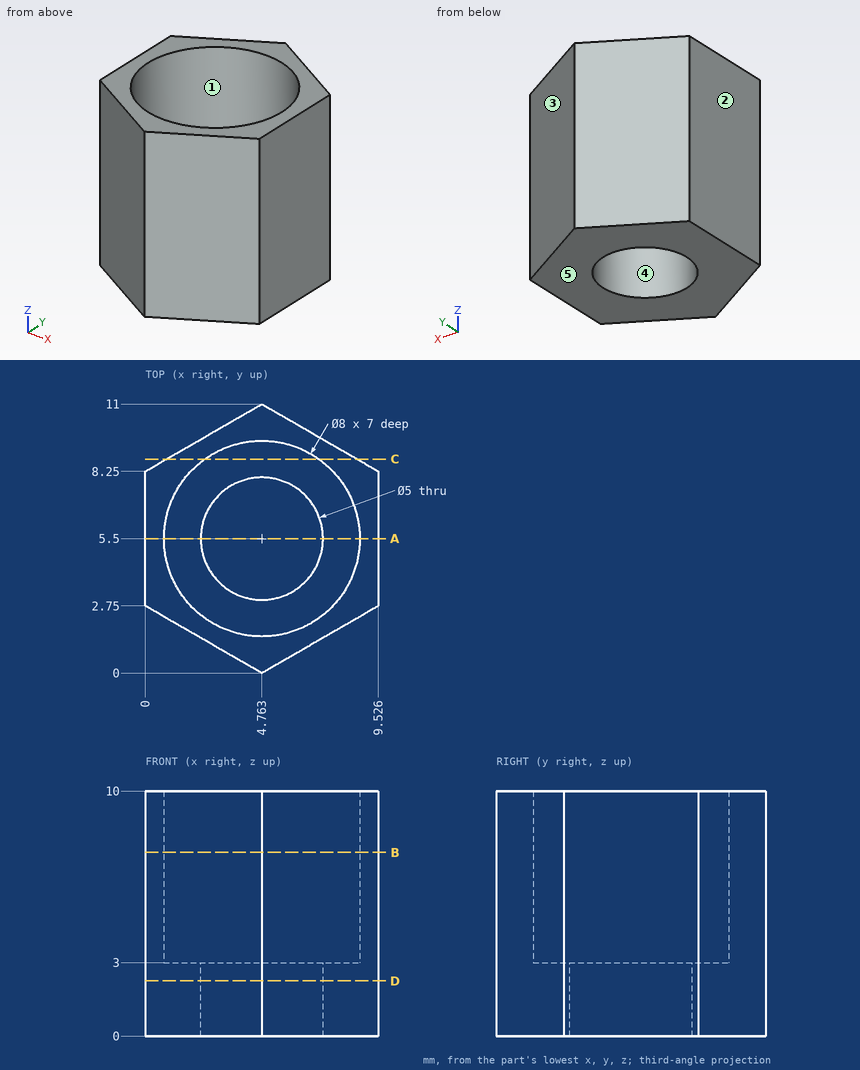
Design review of the part shown in the three views and the two pictorial views. Dimensions are in mm from the part's minimum x, y and z. A direction names the side the tool comes from. Give positions to 0.01 mm unless a question says otherwise; leave off trailing zeros. Write each loop counter-clockwise with the first axis right and the second up, starting at its lowest first coordinate (ties: lowest second). Pieces come first, ordered by that corner, then holes. Notation, with made-up numbers: (-33.5, 11.25) - (18.5, 11.25) arc R13 cw to (18.5, 31.25) - close; hole circle Ø9 at (8, 87.5). An arc over 180 degrees is marked (long way). Return JSON: item names as keys, results as strings. Group by question number.
(1) We need section B-B, the plane z = 7.5. Give the boundary of the cut face in (x, y).
(2) Machinability: for the marked faces 1 and 2, which of the approach directions +Z, -Z, +X, -X, +Y, -Y give a long, thin tool a straight path to every point of the face, cutting with its end or side? Answer none if there is none.
(3) We need section A-A, the plane y = 5.5. Give the boundary of the cut face in (x, z).
(4) Mouldability with a two-part tool opening along Y and no side actions: class the marked faces 3, 4 and 5 as +Y half, -Y half, draft (parallel to the pull), parting line (faces both ways), or undercut.
(5) We need section C-C, the plane y = 8.75. Give the boundary of the cut face in (x, z) (1 decimal).
(6) Insertion check: pin 1 (1 mm diameter, centred on y = 1, z = 4.5, fed in from -X) (1 decimal); pin 2 (1 mm diameter, centred on x = 7.5, y = 5, fed in from +Z); pin 3 (4 mm diameter, centred on x = 4.5, z = 6, fed in from +Y). Each pin has a flat end and moves straight along its axis. Give the tip position at first contact, or say it passes through.
(7) We need section D-D, the plane z = 2.25. Give the boundary of the cut face in (x, y).
(8) To check wall thickness, follow probe 1 along X at (y, z) = (5.5, 0.8); probe 2 along X at (y, z) = (5.5, 6.5); probe 3 along Z at (x, y) = (2.25, 4.25). State the ranges of each line that lie inside material, in increasing order.
Reported:
{
 "1": {"outline": "(0, 2.75) - (4.76, 0) - (9.53, 2.75) - (9.53, 8.25) - (4.76, 11) - (0, 8.25) - close; hole circle Ø8 at (4.76, 5.5)"},
 "2": {"face 1": "+Z", "face 2": "+Z, -Z, -X, +Y, -Y"},
 "3": {"outline": "(0, 0) - (2.26, 0) - (2.26, 3) - (0.76, 3) - (0.76, 10) - (0, 10) - close; (7.26, 0) - (9.53, 0) - (9.53, 10) - (8.76, 10) - (8.76, 3) - (7.26, 3) - close"},
 "4": {"face 3": "+Y half", "face 4": "undercut", "face 5": "draft"},
 "5": {"outline": "(0.9, 0) - (8.7, 0) - (8.7, 10) - (7.1, 10) - (7.1, 3) - (2.4, 3) - (2.4, 10) - (0.9, 10) - close"},
 "6": {"pin 1": "stops at x = 2.2", "pin 2": "stops at z = 3", "pin 3": "stops at y = 11"},
 "7": {"outline": "(0, 2.75) - (4.76, 0) - (9.53, 2.75) - (9.53, 8.25) - (4.76, 11) - (0, 8.25) - close; hole circle Ø5 at (4.76, 5.5)"},
 "8": {"probe 1": "x = 0 to 2.26, 7.26 to 9.53", "probe 2": "x = 0 to 0.76, 8.76 to 9.53", "probe 3": "z = 0 to 3"}
}
